Autodesk Inventor part; units mm, degrees
ref_plane "YZ Plane" through (0, 0, 0) normal (1, 0, 0) x (0, 1, 0)
ref_plane "XZ Plane" through (0, 0, 0) normal (0, 1, 0) x (-1, 0, 0)
ref_plane "XY Plane" through (0, 0, 0) normal (0, 0, 1) x (1, 0, 0)
sketch "Sketch1" plane through (0, 0, 0) normal (0, 1, 0) x (-1, 0, 0)
  arc A0 (-2.1, -2.0718) -> (-2.1, 2.0718) centre (0, 0) ccw
  arc A1 (1, 1.05) -> (1, -1.05) centre (0, 0) ccw
  line L0 (1, 0) -> (1, 1.05)
  line L1 (1, 0) -> (1, -1.05)
  arc A2 (-2.2177, -1.9454) -> (-2.2177, 1.9454) centre (0, 0) ccw
  line L2 (-2.3, -1.8473) -> (-2.3, 1.8473)
  arc A3 (-2.3, -1.8473) -> (-2.3, 1.8473) centre (0, 0) ccw
  dimension "d0" = 5.9
  dimension "d1" = 2.9
  dimension "d2" = 1
  dimension "d7" = 2.3
extrude "Extrusion1" add sketch "Sketch1" along normal blind 5
properties part number "shaft-adapter"
Read the model definition and answer for the solid it produces. Units are mm, in the model's axes. Round coordinates to 2 decimals unless told otherwise and drop trailing zeros. Write each loop counter-clockwise with the first axis right and the second up, starting at its lowest first coordinate (ties: lowest second). Pieces come first, ordered by that corner, then holes.
Q1. The mould has two halves that part along Z. Classify faces 1 (the face through (2.3, 2, 0)), 2 (the face through (-2.95, 2.46, 0.1)), 3 (the face through (-1, 2, 0)): released by +Z, released by -Z, zero draft, split by the parting line, or undercut.
Values:
face 1: zero draft
face 2: split by the parting line
face 3: undercut
Q2. Find section B-B on z = 0. Determine the outline of the cut face in (x, y).
Values:
outline: (-2.95, 0) - (-1, 0) - (-1, 5) - (-2.95, 5) - close; (1.45, 0) - (2.3, 0) - (2.3, 5) - (1.45, 5) - close
Q3. Straight lines are drawn through the part: line 1 (Z direction, x = 0, y = 2.1); line 2 (X direction, y = 2.35, z = 0); line 3 (X direction, y = 1.35, z = -0.8). For each, find the intervals that lie inside material, in ascending order.
Values:
line 1: z = -2.95 to -1.45, 1.45 to 2.95
line 2: x = -2.95 to -1, 1.45 to 2.3
line 3: x = -2.84 to -1, 1.21 to 2.3
Q4. Find section C-C on y = 3.85. Determine the outline of the cut face in (x, z).
Values:
outline: (2.1, -2.07) arc R2.95 ccw to (2.22, -1.95) arc R2.95 ccw to (2.3, -1.85) - (2.3, 1.85) arc R2.95 ccw (long way) to start; hole (-1, -1.05) arc R1.45 ccw (long way) to (-1, 1.05) - close
Q5. Flat-ended cylindrical pins translate along their axes: P1, Ø1.5, axis at x = -2.5, y = 3, coming from the +Z side; P2, Ø1.5, axis at x = -1, y = 3.5, coming from the +Z side. Find the tip coordinate at first contact, or state that the pin passes through.
Values:
P1: stops at z = 2.37
P2: stops at z = 2.94
Q6. Find section A-A on x = 0. Determine the outline of the cut face in (y, z).
Values:
outline: (0, -2.95) - (5, -2.95) - (5, -1.45) - (0, -1.45) - close; (0, 1.45) - (5, 1.45) - (5, 2.95) - (0, 2.95) - close
Q7. Find section D-D on z = -1.55. Determine the outline of the cut face in (x, y), and give its area (3 significant figures).
Values:
outline: (-2.51, 0) - (2.3, 0) - (2.3, 5) - (-2.51, 5) - close
area: 24.0 mm2
